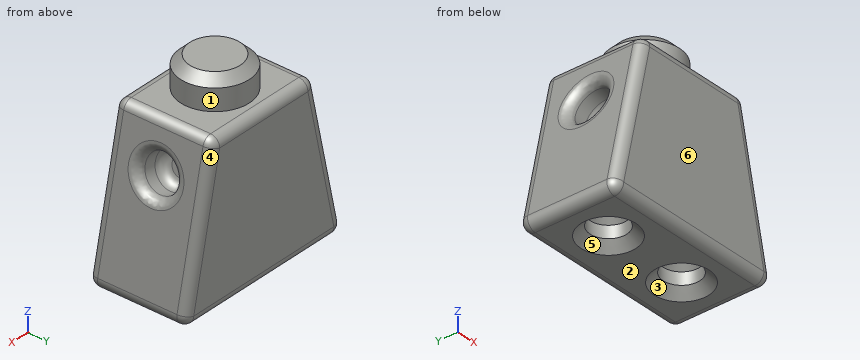
Autodesk Inventor part; units mm, degrees
ref_plane "YZ Plane" through (0, 0, 0) normal (1, 0, 0) x (0, 1, 0)
ref_plane "XZ Plane" through (0, 0, 0) normal (0, 1, 0) x (-1, 0, 0)
ref_plane "XY Plane" through (0, 0, 0) normal (0, 0, 1) x (1, 0, 0)
sketch "Sketch1" plane through (0, 0, 0) normal (0, 1, 0) x (-1, 0, 0)
  line L0 (0, 0) -> (15.44, 0)
  line L1 (2.85, 12.77) -> (12.59, 12.77)
  line L2 (12.59, 12.77) -> (15.44, 0)
  line L3 (2.85, 12.77) -> (0, 0)
  dimension "d0" = 15.44
  dimension "d1" = 9.74
  dimension "d2" = 12.77
extrude "Body" add sketch "Sketch1" along normal blind 8
fillet "Edge" radius 0.75 12 edges at (-12.59, 4, 12.77) (-2.85, 4, 12.77) (0, 4, 0) (-15.44, 4, 0) (-7.72, 0, 0) (-7.72, 8, 0) (-14.015, 0, 6.385) (-7.72, 0, 12.77) (-1.425, 0, 6.385) (-1.425, 8, 6.385) (-7.72, 8, 12.77) (-14.015, 8, 6.385)
sketch "Sketch5" plane through (-11.9889, 0.75, 12.77) normal (0, 0, 1) x (1, 0, 0)
  circle A0 centre (4.2689, 3.25) radius 2.81
  point P0 (11.9889, -0.75)
  dimension "d9" = 5.62
extrude "Head Joint" add sketch "Sketch5" along normal blind 2.5
chamfer "Head Edge" distance 0.75 angle 45 1 edges at (-10.53, 4, 15.27)
sketch "Sketch6" plane through (-0.9358, 0.75, 0) normal (0, 0, -1) x (-1, 0, 0)
  line L0 (13.5683, 6.5) -> (13.5683, 0)
  line L1 (0, 0) -> (0, 6.5)
  circle A0 centre (3.25, 3.25) radius 1.5
  circle A1 centre (10.3183, 3.25) radius 1.5
  point P0 (-0.9358, -0.75)
  dimension "d15" = 3
  dimension "d16" = 3
  dimension "d17" = 3.25
  dimension "d18" = 3.25
extrude "Leg Joint" cut sketch "Sketch6" against normal blind 2.5
chamfer "Leg Edge" distance 0.75 angle 45 4 edges at (-2.6858, 4, 0) (-9.7542, 4, 0) (-9.7542, 4, 2.5) (-2.6858, 4, 2.5)
sketch "Sketch7" plane through (-0.2038, 0.75, 0.9134) normal (0.976, 0, 0.2178) x (0.2178, 0, -0.976)
  line L0 (-11.5473, 0) -> (-11.5473, 6.5)
  circle A0 centre (-8.2973, 3.25) radius 1.5
  point P0 (0.9358, -0.75)
  dimension "d24" = 3
  dimension "d25" = 3.25
extrude "Arm Joint1" cut sketch "Sketch7" against normal blind 2.5
fillet "Arm Edge1" radius 0.75 2 edges at (-4.7798, 4, 9.9304) (-2.3379, 4, 10.4754)
sketch "Sketch8" plane through (-12.7209, 0.75, 12.1834) normal (-0.976, 0, 0.2178) x (0.2178, 0, 0.976)
  line L0 (0, 6.5) -> (0, 0)
  circle A0 centre (-3.25, 3.25) radius 1.5
  point P0 (-9.12, -0.75)
  dimension "d29" = 3
  dimension "d30" = 3.25
extrude "Arm Joint2" cut sketch "Sketch8" against normal blind 2.5
fillet "Arm Edge2" radius 0.75 2 edges at (-13.7556, 4, 7.5474) (-11.3136, 4, 7.0024)
properties part number "Lego Body"
Work out the finished part from the listing and answer in its coordinate system (mm). Face numbers are marked on the shaded views. A direction names the side the tool comes from. Give positions to 0.01 mm unless a question says otherwise; leave off trailing zeros. Loops run counter-clockwise (first coordinate to the right, second up) from the corner with the lowest first, then second, coordinate; pieces in that order, holes last. Notation, with made-up numbers: (-20.5, 70) - (12.5, 70) arc R19 cw to (12.5, 101) - close; hole circle Ø4 at (-26, 86.25). An arc over 180 degrees is marked (long way). Answer in a Markdown table with one row per item. Add a question column.
Q1. The part is cut by section C-C (z = 14). Determine the outline of the cut face in (x, y), and give its area (3 significant figures).
Q2. The part is cut by section B-B (y = 1). Determine the outline of the cut face in (x, z), and give its area (3 significant figures).
Q3. Determine the mould class of the marked faces 3, 4, 5 and 6 for opening direction X: released by +X, released by -X, zero draft, split by the parting line, or undercut.
Q4. Consider line 1 along Z through (x, y) = (-11.5, 2.75); line 2 along Z through (x, y) = (-12.5, 5); line 3 along Z through (x, y) = (-6.75, 1). Determine where each line is inside the solid, lowest interval first.
Q5. Each of these flat-tipped pins is pushed along its axis until it touches: P1, Ø2.5, axis at x = -11.25, y = 4, coming from the +Z side; P2, Ø4, axis at y = 4, z = 10.5, coming from the +X side; P3, Ø1, axis at y = 4.5, z = 2.5, coming from the +X side. Where does it stop, or does it pass through?
Q6. A tool of negligible diameter and unlimited length cuts with its end or side. For the marked faces 1 and 2, from which of +Z, -Z, +X, -X, +Y, -Y can it reach the whole face along a straight path? Write none if from no direction.
Q7. The part is cut by section A-A (x = -7.72). Determine the outline of the cut face in (y, z), and give its area (3 significant figures).
Solution:
| question | item | result |
|---|---|---|
| 1 | outline | circle Ø5.62 at (-7.72, 4) |
| 1 | area | 24.8 mm² |
| 2 | outline | (-15.24, 0.91) arc R0.75 ccw to (-14.5, 0) - (-0.94, 0) arc R0.75 ccw to (-0.2, 0.91) - (-2.72, 12.18) arc R0.75 ccw to (-3.45, 12.77) - (-11.99, 12.77) arc R0.75 ccw to (-12.72, 12.18) - close |
| 2 | area | 160 mm² |
| 3 | face 3 | undercut |
| 3 | face 4 | released by +X |
| 3 | face 5 | undercut |
| 3 | face 6 | zero draft |
| 4 | line 1 | z = 1.98 to 7.93, 9.43 to 12.77 |
| 4 | line 2 | z = 0.65 to 7.66, 9.95 to 12.57 |
| 4 | line 3 | z = 0 to 12.77 |
| 5 | P1 | stops at z = 15.05 |
| 5 | P2 | stops at x = -2.22 |
| 5 | P3 | stops at x = -0.45 |
| 6 | face 1 | +Z |
| 6 | face 2 | -Z, +X, -X, +Y, -Y |
| 7 | outline | (0, 0.75) arc R0.75 ccw to (0.75, 0) - (7.25, 0) arc R0.75 ccw to (8, 0.75) - (8, 12.02) arc R0.75 ccw to (7.25, 12.77) - (6.81, 12.77) - (6.81, 14.52) - (6.06, 15.27) - (1.94, 15.27) - (1.19, 14.52) - (1.19, 12.77) - (0.75, 12.77) arc R0.75 ccw to (0, 12.02) - close |
| 7 | area | 115 mm² |
